```python
from build123d import *

# Parameters (mm, degrees)
CUT_EXTRUDE2_DEPTH = 1.43
FILLET5_R          = 0.3
DRAFT2_ANGLE       = -30


with BuildPart() as part:
    # Sketch1 → Base (revolve)
    with BuildSketch(Plane.XY):
        with BuildLine():
            Line((32.15, 1.5), (3.15, 1.5))
            Line((3.15, 1.5), (2.15, 1.5))
            Line((2.15, 1.5), (2.15, 1.8))
            Line((2.15, 1.8), (2.15, 2.75))
            Line((2.15, 2.75), (0.562803405, 2.75))
            ThreePointArc((0.562803405, 2.75), (0.142144061, 1.403499882), (0, 0))
            Line((0, 0), (32.15, 0))
            Line((32.15, 0), (32.15, 1.5))
        make_face()
    revolve(axis=Axis((4.515812911, 0, 0), (-1, 0, 0)))

    # Sketch6 → Cut-Extrude2 (cut)
    with BuildSketch(Plane(origin=(0, 0, 0), x_dir=(0, 0, -1), z_dir=(1, 0, 0))):
        Polygon((0.35, 0.35), (0.35, 1.75), (-0.35, 1.75), (-0.35, 0.35), (-1.75, 0.35), (-1.75, -0.35), (-0.35, -0.35), (-0.35, -1.75), (0.35, -1.75), (0.35, -0.35), (1.75, -0.35), (1.75, 0.35), align=None)
    extrude(amount=CUT_EXTRUDE2_DEPTH, mode=Mode.SUBTRACT)

    # Fillet5
    fillet5_edges = [part.edges().sort_by_distance(p)[0] for p in [
        (0.723760965, 0.35, 0.35),
        (0.723760965, -0.35, 0.35),
        (0.723760965, -0.35, -0.35),
        (0.723760965, 0.35, -0.35),
    ]]
    fillet(fillet5_edges, radius=FILLET5_R)

    # Draft2
    draft2_faces = [part.faces().sort_by_distance(p)[0] for p in [
        (0.827643319, 0, 1.75),
        (0.827643319, 1.75, 0),
        (0.827643319, -1.75, 0),
        (0.827643319, 0, -1.75),
    ]]
    draft(draft2_faces, Plane(origin=(0, 0, 0), x_dir=(0, 0, 1), z_dir=(1, 0, 0)), DRAFT2_ANGLE)


solid = part.part
```
Verification items for the finished model (mm, model axes). A direction names the side the tool comes from. Round coordinates to 2 decimals unless told otherwise and drop trailing zeros. Order: outer loops, then holes, each group sorted by start corner. A loop starts at its lowest first (then second) coordinate and runs counter-clockwise, first axis right, second up. Notation, with made-up numbers: (-19.5, 81) -> (6.5, 81) arc R15 ccw to (6.5, 89) -> close; hole circle Ø6 at (-20, 47). An arc over 180 degrees is marked (long way). Put each result on its own line as item: value. Start each with the question number.
(1) Draft check along Y on faces 4 (the face through (2.15, -1.2, 1.2)), 5 (the face through (1.345, -0.596, 2.685)), 6 (the face through (0.6, 1, 0.35)). Enter one of: +Y half, -Y half, draft (parallel to the pull), parting line (faces both ways), or undercut.
(2) Material ranges on line 1 along X through (y, z) = (0.05, 0.5); line 2 along X through (y, z) = (-1.55, -1.55); line 3 along Y through (x, z) = (12, 1.35), recorded low to high.
(3) Section check C-C (x = 14). Enter the section's corners in (y, z).
(4) Tool access check on faces 1 (the face through (1.43, 0, 0)), 2 (the face through (32.15, 0, 0)), 3 (the face through (16.94, -1.5, -0.07)). Record the directions out of +Z, -Z, +X, -X, +Y, -Y that give a thin tool (end or side, any length) a straight path to the whole face; none if there is none.
(5) Section check D-D (z = 2.15). Enter the section's corners in (x, y).
(6) Depth check by flat-ended pin: pin 1 Ø1 at (y, z) = (-1, 0) entering from -X; pin 2 Ø1.1 at (x, y) = (1, 1) entering from -Z; pin 3 Ø1.1 at (x, z) = (0.5, -1) entering from +Y. Enter the tip coordinate at first touch or a pass-through.
(7) Section check A-A (z = 0). Enter the section's corners in (x, y), then the cut area to 3 significant figures.
Completed:
1. face 4: draft
1. face 5: parting line
1. face 6: undercut
2. line 1: x = 1.43 to 32.15
2. line 2: x = 0.35 to 2.15
2. line 3: y = -0.65 to 0.65
3. outline: circle Ø3 at (0, 0)
4. face 1: -X
4. face 2: +Z, -Z, +X, +Y, -Y
4. face 3: +X
5. outline: (0.56, -1.71) -> (2.15, -1.71) -> (2.15, 1.71) -> (0.56, 1.71) arc R6.66 ccw to start
6. pin 1: stops at x = 0.04
6. pin 2: stops at z = -2.71
6. pin 3: stops at y = 2.71
7. outline: (0.19, -1.64) arc R7 ccw to (0.56, -2.75) -> (2.15, -2.75) -> (2.15, -1.5) -> (32.15, -1.5) -> (32.15, 1.5) -> (2.15, 1.5) -> (2.15, 2.75) -> (0.56, 2.75) arc R7 ccw to (0.19, 1.64) -> (1.43, 0.92) -> (1.43, -0.92) -> close
7. area: 97.2 mm2
